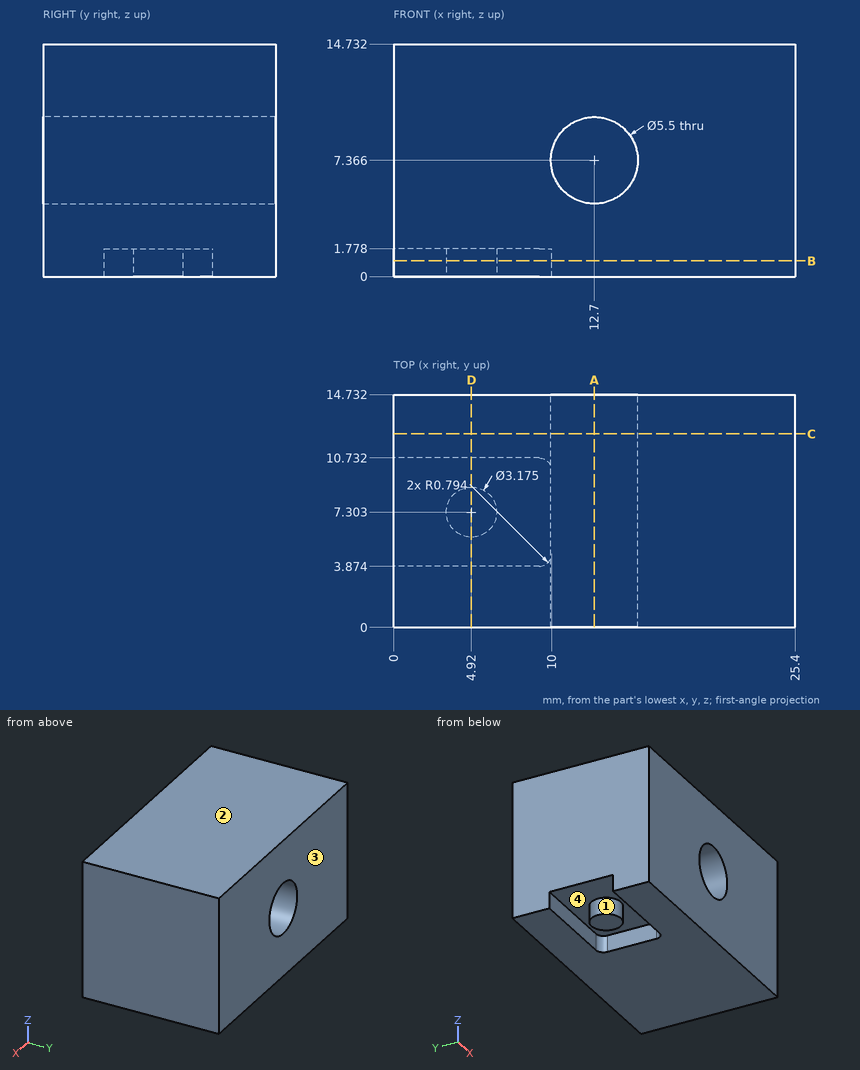
Geometry check sheet. Reference: drawing and pictorial views, mm from the part's lowest x, y, z. Give positions to 0.01 mm unless a question says otherwise; leave off trailing zeros. Loops run counter-clockwise (first coordinate to the right, second up) from the corner with the lowest first, then second, coordinate; pieces in that order, holes last. Notation, with made-up numbers: (7, -6) -> (57, -6) arc R14 cw to (57, 21) -> close; hole circle Ø9 at (-8.75, 18). An arc over 180 degrees is marked (long way). Answer in a Markdown table with one row per item. Add a question column.
1) Cross-section at B-B on z = 1. Record the boundary of the cut face in (x, y) (1 decimal), and give its area (3 significant figures).
2) Cross-section at C-C on y = 12.25. Record the boundary of the cut face in (x, z).
3) Gauge pin test, flat ends, axial feed: P1, Ø0.9, axis at y = 8.5, z = 1, coming from the -X side; P2, Ø3.5, axis at x = 12.7, z = 7.366, coming from the +Y side. Record the tip position at first contact, or that the pin passes through.
4) Cross-section at A-A on x = 12.7. Record the boundary of the cut face in (y, z), and give its area (3 significant figures).
5) Draft check along Y on the marked faces 1, 2, 3 and 4. Enter one of: pulls with the +Y half, pulls with the -Y half, needs draft (parallel to the pull), parting line crosses it, or undercut.
6) Cross-section at D-D on x = 4.92. Record the boundary of the cut face in (y, z) (1 decimal).
7) Material ranges on probe 1 along X at (y, z) = (5, 6); probe 2 along Z at (x, y) = (7, 9); probe 3 along X at (y, z) = (1.5, 8.5) (1 decimal), recorded low to high. Write a range as from..to.
Outcome:
| question | item | result |
|---|---|---|
| 1 | outline | (0, 0) -> (25.4, 0) -> (25.4, 14.7) -> (0, 14.7) -> (0, 10.7) -> (9.2, 10.7) arc R0.8 cw to (10, 9.9) -> (10, 4.7) arc R0.8 cw to (9.2, 3.9) -> (0, 3.9) -> close; circle Ø3.2 at (4.9, 7.3) |
| 1 | area | 314 mm^2 |
| 2 | outline | (0, 0) -> (25.4, 0) -> (25.4, 14.73) -> (0, 14.73) -> close; hole circle Ø5.5 at (12.7, 7.37) |
| 3 | P1 | stops at x = 3.52 |
| 3 | P2 | passes through |
| 4 | outline | (0, 0) -> (14.73, 0) -> (14.73, 4.62) -> (0, 4.62) -> close; (0, 10.12) -> (14.73, 10.12) -> (14.73, 14.73) -> (0, 14.73) -> close |
| 4 | area | 136 mm^2 |
| 5 | face 1 | undercut |
| 5 | face 2 | needs draft |
| 5 | face 3 | pulls with the +Y half |
| 5 | face 4 | undercut |
| 6 | outline | (0, 0) -> (3.9, 0) -> (3.9, 1.8) -> (5.7, 1.8) -> (5.7, 0) -> (8.9, 0) -> (8.9, 1.8) -> (10.7, 1.8) -> (10.7, 0) -> (14.7, 0) -> (14.7, 14.7) -> (0, 14.7) -> close |
| 7 | probe 1 | x = 0..10.31, 15.09..25.4 |
| 7 | probe 2 | z = 1.78..14.73 |
| 7 | probe 3 | x = 0..10.2, 15.2..25.4 |
